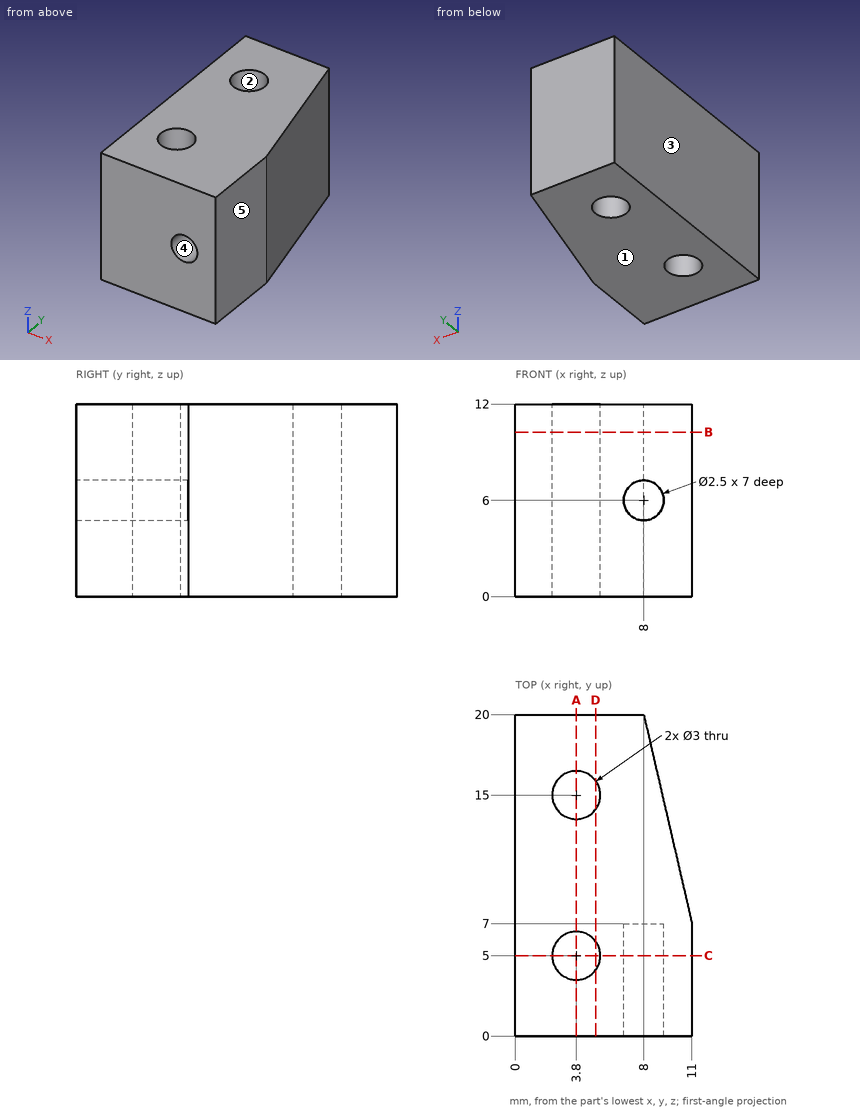
For this review, use the dimensioned drawing (mm, ordinates from the lowest corner) and the shaded views. A direction names the side the tool comes from. Give positions to 0.01 mm unless a question says otherwise; leave off trailing zeros. Write each loop counter-clockwise with the first axis right and the second up, starting at its lowest first coordinate (ties: lowest second). Pieces come first, ordered by that corner, then holes.
(1) Consider section B-B, the plane z = 10.25. Give the boundary of the cut face in (x, y), and give its area (3 significant figures).
(2) Tool access review of the marked faces 4 and 5: name each direction out of +Z, -Z, +X, -X, +Y, -Y from which nothing blocks a thin tool from reaching the whole face with its end or side.
(3) To check wall thickness, follow L1, parallel to Y at x = 3.8, z = 4.75; L2, parallel to X at y = 3.25, z = 6; L3, parallel to Y at x = 4.5, z = 11. State the ranges of each line that lie inside material, in increasing order.
(4) For P1, Ø3, axis at y = 14, z = 1.5, coming from the -X side; P2, Ø0.8, axis at x = 8.5, z = 6, coming from the -Y side, all flat-tipped, find the tip position at first contact; note any pin that passes through.
(5) The part is to be moulded in two halves that separate along X. For the marked faces 1, 2 and 3, say which applies: released by +X, released by -X, zero draft, split by the parting line, or undercut.
(6) Consider section D-D, the plane x = 5. Give the boundary of the cut face in (y, z), and give its area (3 significant figures).
(7) Consider section A-A, the plane x = 3.8. Give the boundary of the cut face in (y, z), and give its area (3 significant figures).
(8) Consider section C-C, the plane y = 5. Give the boundary of the cut face in (x, z).
Returned:
1. outline: (0, 0) - (11, 0) - (11, 7) - (8, 20) - (0, 20) - close; hole circle Ø3 at (3.8, 5); hole circle Ø3 at (3.8, 15)
1. area: 186 mm2
2. face 4: -Y
2. face 5: +Z, -Z, +X, +Y, -Y
3. L1: y = 0 to 3.5, 6.5 to 13.5, 16.5 to 20
3. L2: x = 0 to 6.75, 9.25 to 11
3. L3: y = 0 to 3.67, 6.33 to 13.67, 16.33 to 20
4. P1: stops at x = 0
4. P2: stops at y = 7
5. face 1: zero draft
5. face 2: undercut
5. face 3: released by -X
6. outline: (0, 0) - (4.1, 0) - (4.1, 12) - (0, 12) - close; (5.9, 0) - (14.1, 0) - (14.1, 12) - (5.9, 12) - close; (15.9, 0) - (20, 0) - (20, 12) - (15.9, 12) - close
6. area: 197 mm2
7. outline: (0, 0) - (3.5, 0) - (3.5, 12) - (0, 12) - close; (6.5, 0) - (13.5, 0) - (13.5, 12) - (6.5, 12) - close; (16.5, 0) - (20, 0) - (20, 12) - (16.5, 12) - close
7. area: 168 mm2
8. outline: (0, 0) - (2.3, 0) - (2.3, 12) - (0, 12) - close; (5.3, 0) - (11, 0) - (11, 12) - (5.3, 12) - close; hole circle Ø2.5 at (8, 6)
